For this review, take the finished solid that the model builds, in its own axes (mm). Face numbers are marked on the shaded views. A direction names the side the tool comes from. Give positions to 0.01 mm unless a question says otherwise; leave off trailing zeros. Order: outer loops, then holes, each group sorted by start corner. A loop starts at its lowest first (then second) coordinate and runs counter-clockwise, first axis right, second up.
Autodesk Inventor part; units mm, degrees
ref_plane "YZ Plane" through (0, 0, 0) normal (1, 0, 0) x (0, 1, 0)
ref_plane "XZ Plane" through (0, 0, 0) normal (0, 1, 0) x (-1, 0, 0)
ref_plane "XY Plane" through (0, 0, 0) normal (0, 0, 1) x (1, 0, 0)
sketch "Sketch2" plane through (0, 0, 0) normal (0, 1, 0) x (-1, 0, 0)
  line L0 (0, 0) -> (184.15, 0)
  line L1 (184.15, 0) -> (184.15, -127)
  line L2 (184.15, -127) -> (0, -127)
  line L3 (0, -127) -> (0, 0)
  line L4 (179.07, -121.92) -> (5.08, -121.92)
  line L5 (5.08, -121.92) -> (5.08, -5.08)
  line L6 (5.08, -5.08) -> (179.07, -5.08)
  line L7 (179.07, -5.08) -> (179.07, -121.92)
  dimension "d0" = 184.15
  dimension "d1" = 127
  dimension "d2" = 5.08
  dimension "d3" = 5.08
  dimension "d4" = 5.08
  dimension "d5" = 5.08
extrude "Extrusion1" add sketch "Sketch2" along normal blind 101.6 contours L0 L1 L2 L3 | L4 L5 L6 L7
extrude "Extrusion2" cut sketch "Sketch2" along normal blind 96.52 contours L4 L5 L6 L7
sketch "Sketch3" plane through (-184.15, 0, 0) normal (0, 0, 1) x (1, 0, 0)
  line L0 (184.15, 0) -> (184.15, 101.6)
  line L1 (184.15, 0) -> (0, 0)
  line L2 (0, 0) -> (0, 101.6)
  line L3 (0, 101.6) -> (184.15, 101.6)
  line L4 (184.15, 101.6) -> (184.15, 0)
  dimension "d10" = 184.15
  dimension "d11" = 101.6
extrude "Extrusion3" cut sketch "Sketch3" against normal up to surface (5.08 mm away)
properties part number "Box_Top"
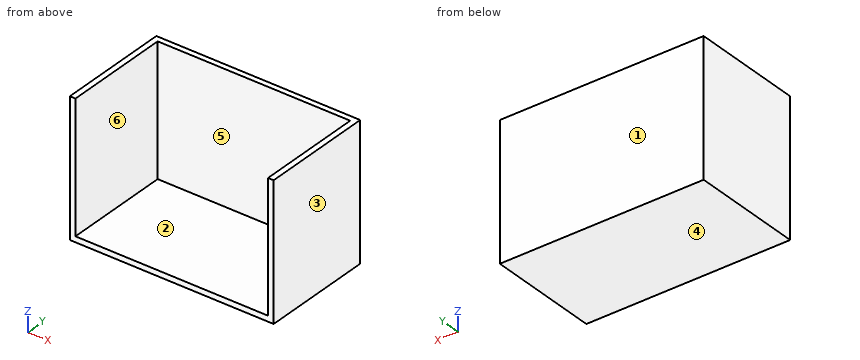
1) We need section B-B on y = 27. Give the boundary of the cut face in (x, z).
Answer sheet:
outline: (-184.15, -127) - (0, -127) - (0, -5.08) - (-5.08, -5.08) - (-5.08, -121.92) - (-179.07, -121.92) - (-179.07, -5.08) - (-184.15, -5.08) - close
2) We need section A-A on z = -106. Give the boundary of the cut face in (x, y), then the cut area to 3 significant figures.
Answer sheet:
outline: (-184.15, 0) - (-179.07, 0) - (-179.07, 96.52) - (-5.08, 96.52) - (-5.08, 0) - (0, 0) - (0, 101.6) - (-184.15, 101.6) - close
area: 1,920 mm2
3) Draft analysis for pull direction X (two halves, no side actions). For the marked faces 3, 4, 5 and 6, state which applies: +X half, -X half, draft (parallel to the pull), parting line (faces both ways), or undercut.
Answer sheet:
face 3: +X half
face 4: draft
face 5: undercut
face 6: undercut
4) We need section C-C on x = -18.5. Give the boundary of the cut face in (y, z).
Answer sheet:
outline: (0, -127) - (101.6, -127) - (101.6, -5.08) - (96.52, -5.08) - (96.52, -121.92) - (0, -121.92) - close
5) Clearance check with flat-ended pins moving along their axes: pin 1 (1 mm diameter, centred on x = -105.5, z = -65.5, fed in from -Y); pin 2 (5 mm diameter, centred on x = -105.5, y = 51.5, fed in from +Z). State where each tip first meets the part, or that it passes through.
Answer sheet:
pin 1: stops at y = 96.52
pin 2: stops at z = -121.92
6) To check wall thickness, follow line 1 (X direction, y = 64, z = -32.5); line 2 (Y direction, x = -8.5, z = -66); line 3 (Z direction, x = -42, y = 9). State the ranges of each line that lie inside material, in increasing order.
Answer sheet:
line 1: x = -184.15 to -179.07, -5.08 to 0
line 2: y = 96.52 to 101.6
line 3: z = -127 to -121.92
7) Tool access review of the marked faces 1 and 2: name each direction out of +Z, -Z, +X, -X, +Y, -Y from which nothing blocks a thin tool from reaching the whole face with its end or side.
Answer sheet:
face 1: +Z, -Z, +X, -X, +Y
face 2: +Z, -Y
